```python
from build123d import *

# Parameters (mm, degrees)
F0_R      = 25.4
F0_R_2    = 7.62
F1_DEPTH  = 127
F0_R_3    = 22.86
F2_DEPTH  = 101.6
F4_DEPTH  = 12.7
F5_W      = 60.96
F5_H      = 60.96
F6_DEPTH  = 50.8
F7_R      = 5.08
F8_SIZE   = 2.54
F9_R      = 27.94
F9_R_2    = 22.86
F10_DEPTH = 12.7
F11_SIZE  = 5.08
F12_SIZE  = 2.54
F13_SIZE  = 2.54
F14_SIZE  = 2.54


with BuildPart() as f1:
    # F0 (on Top) → F1 (new body)
    with BuildSketch(Plane.XY):
        Circle(F0_R)
        Circle(F0_R_2, mode=Mode.SUBTRACT)
    extrude(amount=F1_DEPTH)



with BuildPart() as f2:
    # F0 (on Top) → F2 (new body)
    with BuildSketch(Plane.XY):
        with Locations((101.6, 0)):
            Circle(F0_R_3)
        with Locations((101.6, 0)):
            Circle(F0_R_2, mode=Mode.SUBTRACT)
    extrude(amount=F2_DEPTH)


with BuildPart() as f1_1:
    add(f1.part)

    add(f2.part)  # F4 merges F2
    # F3 (on Front) → F4 (join, symmetric)
    with BuildSketch(Plane.XZ):
        with BuildLine():
            Line((20.32, 127), (20.32, 0))
            Line((20.32, 0), (81.28, 0))
            Line((81.28, 0), (81.28, 81.28))
            ThreePointArc((81.28, 81.28), (61.5844056789, 108.82076155), (33.02, 127))
            Line((33.02, 127), (20.32, 127))
        make_face()
        with BuildLine():
            ThreePointArc((31.63198664, 113.8086976228), (54.1219978961, 98.3677847047), (69.73198664, 75.9947954215))
            Line((69.73198664, 75.9947954215), (69.73198664, 50.3086976228))
            Line((69.73198664, 50.3086976228), (31.63198664, 50.3086976228))
            Line((31.63198664, 50.3086976228), (31.63198664, 113.8086976228))
        make_face(mode=Mode.SUBTRACT)
    extrude(amount=F4_DEPTH, both=True)

    # F5 (on Front) → F6 (cut, symmetric)
    with BuildSketch(Plane.XZ):
        with Locations((-2.54, 55.88)):
            Rectangle(F5_W, F5_H)
    extrude(amount=F6_DEPTH, both=True, mode=Mode.SUBTRACT)

    # F7
    f7_edges = [f1_1.edges().sort_by_distance(p)[0] for p in [
        (31.631987, 0, 50.308698),
        (31.631987, 0, 113.808698),
        (69.731987, 0, 50.308698),
        (69.731987, 0, 75.994795),
    ]]
    fillet(f7_edges, radius=F7_R)

    # F8
    f8_edges = [f1_1.edges().sort_by_distance(p)[0] for p in [
        (-25.4, 0, 127),
        (-25.4, 0, 0),
        (-7.62, 0, 86.36),
        (-7.62, 0, 25.4),
    ]]
    chamfer(f8_edges, length=F8_SIZE)

    # F9 (on Top) → F10 (join)
    with BuildSketch(Plane.XY):
        with Locations((101.6, 0)):
            Circle(F9_R)
        with Locations((101.6, 0)):
            Circle(F9_R_2, mode=Mode.SUBTRACT)
    extrude(amount=F10_DEPTH)

    # F11
    f11_edges = [f1_1.edges().sort_by_distance(p)[0] for p in [
        (93.98, 0, 0),
    ]]
    chamfer(f11_edges, length=F11_SIZE)

    # F12
    f12_edges = [f1_1.edges().sort_by_distance(p)[0] for p in [
        (93.98, 0, 101.6),
    ]]
    chamfer(f12_edges, length=F12_SIZE)

    # F13
    f13_edges = [f1_1.edges().sort_by_distance(p)[0] for p in [
        (129.54, 0, 12.7),
        (129.54, 0, 0),
    ]]
    chamfer(f13_edges, length=F13_SIZE)

    # F14
    f14_edges = [f1_1.edges().sort_by_distance(p)[0] for p in [
        (-7.62, 0, 127),
    ]]
    chamfer(f14_edges, length=F14_SIZE)


solid = f1_1.part
```
Work out the finished part from the listing and answer in its coordinate system (mm). A direction names the side the tool comes from. Give positions to 0.01 mm unless a question says otherwise; leave off trailing zeros. Loops run counter-clockwise (first coordinate to the right, second up) from the corner with the lowest first, then second, coordinate; pieces in that order, holes last. Notation, with made-up numbers: (41.25, 8) -> (91.25, 8) arc R20 cw to (91.25, 37) -> close; hole circle Ø7 at (23.25, 42.5). An arc over 180 degrees is marked (long way). Write item = value, one per line. Start each with the question number.
(1) Find section A-A on z = 103.5. Give the vertices of the cut face in (x, y).
(2) Find section C-C on z = 38. Give the vertices of the cut face in (x, y).
(3) Find section B-B on x = 0. Give the vertices of the cut face in (y, z).
(4) The mould has two halves that part along Y. Classify faces 1 (the flat face through (27.94, 0, 55)), 2 (the cylindrical face through (129.52, -1.04, 6.3)), 3 (the conical face through (-6.14, 4.71, 88.78)): +Y half, -Y half, draft (parallel to the pull), parting line (faces both ways), or undercut.
(5) Which of the six approach directions +Z, -Z, +X, -X, +Y, -Y give full straight-line access (tool end or side, diameter ignored) to faces 4 (the flat face through (69.732, 0, 65)), 5 (the flat face through (123, 10, 12.7)), 6 (the conical face through (-6.14, 4.71, 22.98)), 7 (the cylindrical face through (93.987, 0.335, 51.412)), 8 (the flat face through (106, -10, 101.6))?
(6) Given pin 1 Ø12 at (x, y) = (93, 15) entering from +Z; pin 2 Ø5 at (y, z) = (-12.5, 46) entering from -X; pin 3 Ø2.5 at (y, z) = (11.5, 50.5) entering from +X; pin 4 Ø6 at (x, z) = (35.5, 105) entering from -Y, each flat-ended and moving along its own axis, determine where each tip first touches the part or whether it passes through.
(7) Find section D-D on x = 101.6. Give the vertices of the cut face in (y, z), and give its area (3 significant figures).
(8) Find the intervals of material crossed by probe 1 along X at (y, z) = (-12, 74.5); probe 2 along X at (y, z) = (-3.5, 23); probe 3 along Y at (x, z) = (101.6, 31), in increasing order. Write a range as from..to.
From the geometry:
q1.outline = (22, -12.7) -> (31.63, -12.7) -> (31.63, 12.7) -> (22, 12.7) arc R25.4 ccw (long way) to start; (48.4, -12.7) -> (66.75, -12.7) -> (66.75, 12.7) -> (48.4, 12.7) -> close; hole circle Ø15.24 at (0, 0)
q2.outline = (27.94, -12.7) -> (81.28, -12.7) -> (81.28, -10.47) arc R22.86 ccw (long way) to (81.28, 10.47) -> (81.28, 12.7) -> (27.94, 12.7) -> close; hole circle Ø15.24 at (101.6, 0)
q3.outline = (-25.4, 2.54) -> (-22.86, 0) -> (-7.62, 0) -> (-7.62, 22.86) -> (-10.16, 25.4) -> (-25.4, 25.4) -> close; (-25.4, 86.36) -> (-10.16, 86.36) -> (-7.62, 88.9) -> (-7.62, 124.46) -> (-10.16, 127) -> (-22.86, 127) -> (-25.4, 124.46) -> close; (7.62, 0) -> (22.86, 0) -> (25.4, 2.54) -> (25.4, 25.4) -> (10.16, 25.4) -> (7.62, 22.86) -> close; (7.62, 88.9) -> (10.16, 86.36) -> (25.4, 86.36) -> (25.4, 124.46) -> (22.86, 127) -> (10.16, 127) -> (7.62, 124.46) -> close
q4.face_1 = draft
q4.face_2 = parting line
q4.face_3 = undercut
q5.face_4 = +Y, -Y
q5.face_5 = +Z
q5.face_6 = none
q5.face_7 = +Z, -Z
q5.face_8 = +Z, +X, +Y, -Y
q6.pin_1 = 101.6
q6.pin_2 = 27.94
q6.pin_3 = 122.03
q6.pin_4 = through
q7.outline = (-27.94, 2.54) -> (-25.4, 0) -> (-12.7, 0) -> (-7.62, 5.08) -> (-7.62, 99.06) -> (-10.16, 101.6) -> (-22.86, 101.6) -> (-22.86, 12.7) -> (-25.4, 12.7) -> (-27.94, 10.16) -> close; (7.62, 5.08) -> (12.7, 0) -> (25.4, 0) -> (27.94, 2.54) -> (27.94, 10.16) -> (25.4, 12.7) -> (22.86, 12.7) -> (22.86, 101.6) -> (10.16, 101.6) -> (7.62, 99.06) -> close
q7.area = 3,180 mm^2
q8.probe_1 = 27.94..31.63, 69.73..81.28, 82.14..121.06
q8.probe_2 = -25.16..-6.93, 6.93..94.83, 108.37..124.19
q8.probe_3 = -22.86..-7.62, 7.62..22.86
